```python
from build123d import *

# Parameters (mm, degrees)
F0_W     = 30
F0_H     = 8
F0_R     = 1.7
F1_DEPTH = 6
F2_W     = 8
F2_H     = 8
F2_R     = 1.7
F3_DEPTH = 2
F4_R     = 3.99999


# Not quite as in the source:
# - a fillet or chamfer is up to 0.001 mm smaller than in the source, because OpenCascade refuses the exact size


with BuildPart() as f1:
    # F0 (on Top) → F1 (new body)
    with BuildSketch(Plane.XY):
        Rectangle(F0_W, F0_H)
        with Locations((-11, 0)):
            Circle(F0_R, mode=Mode.SUBTRACT)
        with Locations((11, 0)):
            Circle(F0_R, mode=Mode.SUBTRACT)
    extrude(amount=F1_DEPTH)

    # F2 (on face) → F3 (join)
    with BuildSketch(Plane.XY.offset(6)):
        with Locations((-11, 0)):
            Rectangle(F2_W, F2_H)
        with Locations((-11, 0)):
            Circle(F2_R, mode=Mode.SUBTRACT)
    extrude(amount=F3_DEPTH)

    # F4 (radius 4 in the source; OpenCascade refuses exactly that, so slightly less here)
    f4_edges = [f1.edges().sort_by_distance(p)[0] for p in [
        (-15, 4, 4),
        (-15, -4, 4),
        (15, 4, 3),
        (15, -4, 3),
        (-7, -4, 7),
        (-7, 4, 7),
    ]]
    fillet(f4_edges, radius=F4_R)


solid = f1.part
```
Could you check a few things on this model? Use its own coordinates, in mm. A direction names the side the tool comes from. Round coordinates to 2 decimals unless told otherwise and drop trailing zeros. Order: outer loops, then holes, each group sorted by start corner. A loop starts at its lowest first (then second) coordinate and runs counter-clockwise, first axis right, second up. Notation, with made-up numbers: M 88,81.25 L 102,81.25 A20 ccw 102,97.25 Z; hole C -30,-19.75 d8. An arc over 180 degrees is marked long. One line per question, with ' | ' between items. Start each with the question number.
(1) For P1, Ø4, axis at x = 4.5, y = 1.5, coming from the +Z side; P2, Ø3, axis at y = 3, z = 1.5, coming from the +X side; P3, Ø2, axis at x = -11, y = 0, coming from the +Z side, each with a flat end and sliding along its axis, tell me the tip position at first contact or that it passes through.
(2) Thinking about a two-plate mould opening in X: for faces 1 (the face through (-9.43, -0.65, 3.94)), 2 (the face through (13.797, -2.859, 3.042)), 3 (the face through (0, -4, 3)), which applies, +X half, -X half, draft (parallel to the pull), parting line (faces both ways), or undercut?
(3) For faces 4 (the face through (0, 0, 0)), 5 (the face through (-8.203, -2.859, 7.014)), 6 (the face through (-8.141, 2.797, 7.014)), which set-ups out of +Z, -Z, +X, -X, +Y, -Y let a thin tool reach every point of the face, with its end or its side?
(4) Please list where these lines run through material, in increasing order: line 1 along Y through (x, z) = (-11, 6); line 2 along X through (y, z) = (1.25, 4.5); line 3 along Z through (x, y) = (-4.75, 2).
(5) Suppose I cut it at C-C on y = 1.25. List the corners of the cut face in (x, z) for me.
(6) Suppose I cut it at D-D on x = 1.5. List the corners of the cut face in (y, z) for me.
(7) Suppose I cut it at A-A on z = 3.25. Count the separate pieces of the cut face and the enclosed holes in it, then the cut area to 3 significant figures.
Geometry results:
1) P1: z = 6 | P2: x = 14.71 | P3: through
2) face 1: undercut | face 2: +X half | face 3: draft
3) face 4: -Z, +X, -X, +Y, -Y | face 5: +Z, +X, -Y | face 6: +Z, +X, +Y
4) line 1: -4 to -1.7, 1.7 to 4 | line 2: -14.8 to -12.15, -9.85 to 9.85, 12.15 to 14.8 | line 3: 0 to 6
5) outline: M -14.8,0 L -12.15,0 L -12.15,8 L -14.8,8 Z; M -9.85,0 L 9.85,0 L 9.85,6 L -7.2,6 L -7.2,8 L -9.85,8 Z; M 12.15,0 L 14.8,0 L 14.8,6 L 12.15,6 Z
6) outline: M -4,0 L 4,0 L 4,6 L -4,6 Z
7) separate pieces: 1 | enclosed holes: 2 | area: 208 mm²
